The model under review builds one solid part; all positions refer to its coordinate system, in mm. Coordinates: 2 decimals unless noted, no trailing zeros. Order: outer loops, then holes, each group sorted by start corner. A loop starts at its lowest first (then second) coordinate and runs counter-clockwise, first axis right, second up. Notation, with made-up numbers: (62, 75.5) -> (85, 75.5) arc R18 cw to (85, 84.5) -> close; hole circle Ø1 at (-33, -7.75). An arc over 180 degrees is marked (long way). Use one line per item in the form item = value. Start each with the question number.
(1) Take a section at C-C (y = -2.1). State how many separate pieces and enclosed holes the cut face has, then the cut area to 3 significant figures.
(2) Wall thickness on line 1 along Z through (x, y) = (140, -1.55); line 2 along X through (y, z) = (-4.35, 438.5); line 3 along X through (y, z) = (-2, 253): over which ranges is each line inside the solid? List them lowest first.
(3) Take a section at A-A (z = 260). State the section outline as (x, y) points.
(4) Take a section at B-B (x = 280). State the section outline as (y, z) points.
```python
from build123d import *

# Parameters (mm, degrees)
F0_W     = 404
F0_H     = 510
F0_W_2   = 84.9999959469
F0_H_2   = 127.9999959469
F0_W_3   = 128
F0_H_3   = 85
F0_W_4   = 128.0000081062
F0_H_4   = 85.0000081062
F0_W_5   = 85
F0_H_5   = 128
F1_DEPTH = 5
F2_R     = 2


with BuildPart() as f1:
    # F0 (on Front) → F1 (new body)
    with BuildSketch(Plane.XZ):
        with Locations((202, 255)):
            Rectangle(F0_W, F0_H)
        Polygon((37.5742387427, 29.3041344952), (42.5255790864, 30), (43.917310096, 20.0973193126), (38.9659697523, 19.4014538078), align=None, mode=Mode.SUBTRACT)
        Polygon((28.6082689904, 129.0268068742), (30, 119.1241261867), (25.0486596563, 118.4282606819), (23.6569286467, 128.3309413694), align=None, mode=Mode.SUBTRACT)
        Polygon((168.082689904, 20.0973193126), (169.4744209136, 30), (174.4257612573, 29.3041344952), (173.0340302477, 19.4014538078), align=None, mode=Mode.SUBTRACT)
        Polygon((42.5255790864, 30), (30, 30), (30, 119.1241261867), (30, 139), (182, 139), (182, 119.1241261867), (182, 30), (169.4744209136, 30), align=None, mode=Mode.SUBTRACT)
        Polygon((186.9513403437, 118.4282606819), (182, 119.1241261867), (183.3917310096, 129.0268068742), (188.3430713533, 128.3309413694), align=None, mode=Mode.SUBTRACT)
        Polygon((59.0742387427, 178.3041344952), (64.0255790864, 179), (65.417310096, 169.0973193126), (60.4659697523, 168.4014538078), align=None, mode=Mode.SUBTRACT)
        Polygon((146.582689904, 169.0973193126), (147.9744209136, 179), (152.9257612573, 178.3041344952), (151.5340302477, 168.4014538078), align=None, mode=Mode.SUBTRACT)
        Polygon((229.5742387427, 29.3041344952), (234.5255790864, 30), (235.917310096, 20.0973193126), (230.9659697523, 19.4014538078), align=None, mode=Mode.SUBTRACT)
        Polygon((220.6082689904, 129.0268068742), (222, 119.1241261867), (217.0486596563, 118.4282606819), (215.6569286467, 128.3309413694), align=None, mode=Mode.SUBTRACT)
        Polygon((234.5255790864, 30), (222, 30), (222, 119.1241261867), (222, 139), (374, 139), (374, 119.1241261867), (374, 30), (361.4744209136, 30), align=None, mode=Mode.SUBTRACT)
        Polygon((360.082689904, 20.0973193126), (361.4744209136, 30), (366.4257612573, 29.3041344952), (365.0340302477, 19.4014538078), align=None, mode=Mode.SUBTRACT)
        Polygon((378.9513403437, 118.4282606819), (374, 119.1241261867), (375.3917310096, 129.0268068742), (380.3430713533, 128.3309413694), align=None, mode=Mode.SUBTRACT)
        Polygon((251.0742387427, 178.3041344952), (256.0255790864, 179), (257.417310096, 169.0973193126), (252.4659697523, 168.4014538078), align=None, mode=Mode.SUBTRACT)
        Polygon((338.582689904, 169.0973193126), (339.9744209136, 179), (344.9257612573, 178.3041344952), (343.5340302477, 168.4014538078), align=None, mode=Mode.SUBTRACT)
        Polygon((50.1082689904, 278.0268068742), (51.5, 268.1241261867), (46.5486596563, 267.4282606819), (45.1569286467, 277.3309413694), align=None, mode=Mode.SUBTRACT)
        Polygon((37.5742387427, 370.3041344952), (42.5255790864, 371), (43.917310096, 361.0973193126), (38.9659697523, 360.4014538078), align=None, mode=Mode.SUBTRACT)
        Polygon((64.0255790864, 179), (51.5, 179), (51.5, 268.1241261867), (51.5, 331), (160.5, 331), (160.5, 268.1241261867), (160.5, 179), (147.9744209136, 179), align=None, mode=Mode.SUBTRACT)
        Polygon((165.4513403437, 267.4282606819), (160.5, 268.1241261867), (161.8917310096, 278.0268068742), (166.8430713533, 277.3309413694), align=None, mode=Mode.SUBTRACT)
        Polygon((168.082689904, 361.0973193126), (169.4744209136, 371), (174.4257612573, 370.3041344952), (173.0340302477, 360.4014538078), align=None, mode=Mode.SUBTRACT)
        Polygon((28.6082689904, 470.0268068742), (30, 460.1241261867), (25.0486596563, 459.4282606819), (23.6569286467, 469.3309413694), align=None, mode=Mode.SUBTRACT)
        Polygon((42.5255790864, 371), (30, 371), (30, 460.1241261867), (30, 480), (182, 480), (182, 460.1241261867), (182, 371), (169.4744209136, 371), align=None, mode=Mode.SUBTRACT)
        Polygon((186.9513403437, 459.4282606819), (182, 460.1241261867), (183.3917310096, 470.0268068742), (188.3430713533, 469.3309413694), align=None, mode=Mode.SUBTRACT)
        Polygon((242.1082689904, 278.0268068742), (243.5, 268.1241261867), (238.5486596563, 267.4282606819), (237.1569286467, 277.3309413694), align=None, mode=Mode.SUBTRACT)
        Polygon((256.0255790864, 179), (243.5, 179), (243.5, 268.1241261867), (243.5, 331), (352.5, 331), (352.5, 268.1241261867), (352.5, 179), (339.9744209136, 179), align=None, mode=Mode.SUBTRACT)
        Polygon((229.5742387427, 370.3041344952), (234.5255790864, 371), (235.917310096, 361.0973193126), (230.9659697523, 360.4014538078), align=None, mode=Mode.SUBTRACT)
        Polygon((357.4513403437, 267.4282606819), (352.5, 268.1241261867), (353.8917310096, 278.0268068742), (358.8430713533, 277.3309413694), align=None, mode=Mode.SUBTRACT)
        Polygon((360.082689904, 361.0973193126), (361.4744209136, 371), (366.4257612573, 370.3041344952), (365.0340302477, 360.4014538078), align=None, mode=Mode.SUBTRACT)
        Polygon((234.5255790864, 371), (222, 371), (222, 460.1241261867), (222, 480), (374, 480), (374, 460.1241261867), (374, 371), (361.4744209136, 371), align=None, mode=Mode.SUBTRACT)
        Polygon((220.6082689904, 470.0268068742), (222, 460.1241261867), (217.0486596563, 459.4282606819), (215.6569286467, 469.3309413694), align=None, mode=Mode.SUBTRACT)
        Polygon((378.9513403437, 459.4282606819), (374, 460.1241261867), (375.3917310096, 470.0268068742), (380.3430713533, 469.3309413694), align=None, mode=Mode.SUBTRACT)
        Polygon((51.5, 268.1241261867), (51.5, 179), (64.0255790864, 179), (147.9744209136, 179), (160.5, 179), (160.5, 268.1241261867), (160.5, 331), (51.5, 331), align=None)
        with Locations((106, 255)):
            Rectangle(F0_W_2, F0_H_2, mode=Mode.SUBTRACT)
        Polygon((30, 119.1241261867), (30, 30), (42.5255790864, 30), (169.4744209136, 30), (182, 30), (182, 119.1241261867), (182, 139), (30, 139), align=None)
        with Locations((106, 84.5)):
            Rectangle(F0_W_3, F0_H_3, mode=Mode.SUBTRACT)
        Polygon((222, 119.1241261867), (222, 30), (234.5255790864, 30), (361.4744209136, 30), (374, 30), (374, 119.1241261867), (374, 139), (222, 139), align=None)
        with Locations((298, 84.5)):
            Rectangle(F0_W_4, F0_H_4, mode=Mode.SUBTRACT)
        Polygon((243.5, 268.1241261867), (243.5, 179), (256.0255790864, 179), (339.9744209136, 179), (352.5, 179), (352.5, 268.1241261867), (352.5, 331), (243.5, 331), align=None)
        with Locations((298, 255)):
            Rectangle(F0_W_5, F0_H_5, mode=Mode.SUBTRACT)
        Polygon((30, 460.1241261867), (30, 371), (42.5255790864, 371), (169.4744209136, 371), (182, 371), (182, 460.1241261867), (182, 480), (30, 480), align=None)
        with Locations((106, 425.5)):
            Rectangle(F0_W_3, F0_H_3, mode=Mode.SUBTRACT)
        Polygon((222, 460.1241261867), (222, 371), (234.5255790864, 371), (361.4744209136, 371), (374, 371), (374, 460.1241261867), (374, 480), (222, 480), align=None)
        with Locations((298, 425.5)):
            Rectangle(F0_W_3, F0_H_3, mode=Mode.SUBTRACT)
    extrude(amount=F1_DEPTH)

    # F2
    f2_edges = [f1.edges().sort_by_distance(p)[0] for p in [
        (0, -2.5, 510),
        (404, -2.5, 510),
        (0, -2.5, 0),
        (404, -2.5, 0),
        (233.999996, -2.5, 127.000004),
        (255.5, -2.5, 319),
        (63.500002, -2.5, 318.999998),
        (42, -2.5, 127),
        (234, -2.5, 468),
        (42, -2.5, 468),
        (170, -2.5, 468),
        (362, -2.5, 468),
        (340.5, -2.5, 319),
        (148.499998, -2.5, 318.999998),
        (170, -2.5, 127),
        (362.000004, -2.5, 127.000004),
        (362.000004, -2.5, 41.999996),
        (170, -2.5, 42),
        (148.499998, -2.5, 191.000002),
        (340.5, -2.5, 191),
        (170, -2.5, 383),
        (362, -2.5, 383),
        (42, -2.5, 42),
        (233.999996, -2.5, 41.999996),
        (255.5, -2.5, 191),
        (63.500002, -2.5, 191.000002),
        (42, -2.5, 383),
        (234, -2.5, 383),
    ]]
    fillet(f2_edges, radius=F2_R)


solid = f1.part
```
Findings:
q1.separate_pieces = 1
q1.enclosed_holes = 30
q1.area = 140,000 mm²
q2.line_1 = 0 to 42, 127 to 191, 319 to 383, 468 to 510
q2.line_2 = 0 to 42, 170 to 234, 362 to 404
q2.line_3 = 0 to 63.5, 148.5 to 255.5, 340.5 to 404
q3.outline = (0, -5) -> (63.5, -5) -> (63.5, 0) -> (0, 0) -> close; (148.5, -5) -> (255.5, -5) -> (255.5, 0) -> (148.5, 0) -> close; (340.5, -5) -> (404, -5) -> (404, 0) -> (340.5, 0) -> close
q4.outline = (-5, 0) -> (0, 0) -> (0, 42) -> (-5, 42) -> close; (-5, 127) -> (0, 127) -> (0, 191) -> (-5, 191) -> close; (-5, 319) -> (0, 319) -> (0, 383) -> (-5, 383) -> close; (-5, 468) -> (0, 468) -> (0, 510) -> (-5, 510) -> close
